Work out the finished part from the listing and answer in its coordinate system (mm). Coordinates: 2 decimals unless noted, no trailing zeros. Loops run counter-clockwise (first coordinate to the right, second up) from the corner with the lowest first, then second, coordinate; pieces in that order, holes last. Notation, with made-up numbers: (-27.5, 85.25) - (30.5, 85.25) arc R29 cw to (30.5, 120.25) - close; hole circle Ø3 at (87.25, 59.5). An arc over 180 degrees is marked (long way). Write each question's results on one line, items separated by ' | '. Start each with the question number.
Item 1: Section B-B, the plane x = 53 is taken. Write down the section's boundary in (y, z), plus the area to 3 significant figures.
Item 2: Each of these flat-tipped pins is pushed along its axis until it touches: pin 1 Ø3.5 at (x, z) = (21.35, -38.1) entering from -Y; pin 2 Ø3 at (y, z) = (2, -113) entering from +X. Where does it stop, or does it pass through?
Item 3: Consider probe 1 along Z at (x, y) = (42, 0.5) (3 decimals); probe 2 along Z at (x, y) = (40.4, 4.5) (3 decimals); probe 3 along X at (y, z) = (4, -38.1). Determine where each line is inside the solid, lowest interval first. Write a range as [from, to].
Item 4: Section A-A, the plane z = -337.5 is taken. Write down the section's boundary in (x, y).
from build123d import *

# Parameters (mm, degrees)
BOSS_EXTRUDE1_DEPTH          = 6.35
F_4_0_4_DIAMETER_HOLE1_D     = 4
F_4_0_4_DIAMETER_HOLE1_DEPTH = 10
F_4_0_4_DIAMETER_HOLE1_TIP   = 1.201721238
F_4_0_4_DIAMETER_HOLE2_D     = 4
F_4_0_4_DIAMETER_HOLE2_DEPTH = 10
F_4_0_4_DIAMETER_HOLE2_TIP   = 1.201721238


with BuildPart() as part:
    # Sketch1 → Boss-Extrude1 (new body)
    with BuildSketch(Plane(origin=(0, 0, 0), x_dir=(1, 0, 0), z_dir=(0, 1, 0))):
        Polygon((0, 0), (216.51, 0), (0, 375), align=None)
    extrude(amount=BOSS_EXTRUDE1_DEPTH)

    # Ø4.0 (4) Diameter Hole1
    with Locations(Plane(origin=(31.757248956, 6.35, -326.345678088), x_dir=(0.50000632, 0, 0.866021755), z_dir=(0, 1, 0))):
        with Locations((21.272379971, -34.925), (40.322379971, -12.7), (244.423337674, -153.137564848), (273.195791575, -147.752490889)):
            Hole(F_4_0_4_DIAMETER_HOLE1_D / 2, depth=F_4_0_4_DIAMETER_HOLE1_DEPTH)
            with Locations((0, 0, -(F_4_0_4_DIAMETER_HOLE1_DEPTH + F_4_0_4_DIAMETER_HOLE1_TIP / 2))):  # 118° drill point
                Cone(0, F_4_0_4_DIAMETER_HOLE1_D / 2, F_4_0_4_DIAMETER_HOLE1_TIP, mode=Mode.SUBTRACT)

    # Ø4.0 (4) Diameter Hole2
    with Locations(Plane(origin=(31.757248956, 0, -326.345678088), x_dir=(-0.50000632, 0, -0.866021755), z_dir=(0, -1, 0))):
        with Locations((-21.272379971, -12.7), (-40.322379971, -34.925), (-253.948458076, -136.639850421), (-263.670671173, -164.250205317)):
            Hole(F_4_0_4_DIAMETER_HOLE2_D / 2, depth=F_4_0_4_DIAMETER_HOLE2_DEPTH)
            with Locations((0, 0, -(F_4_0_4_DIAMETER_HOLE2_DEPTH + F_4_0_4_DIAMETER_HOLE2_TIP / 2))):  # 118° drill point
                Cone(0, F_4_0_4_DIAMETER_HOLE2_D / 2, F_4_0_4_DIAMETER_HOLE2_TIP, mode=Mode.SUBTRACT)


solid = part.part
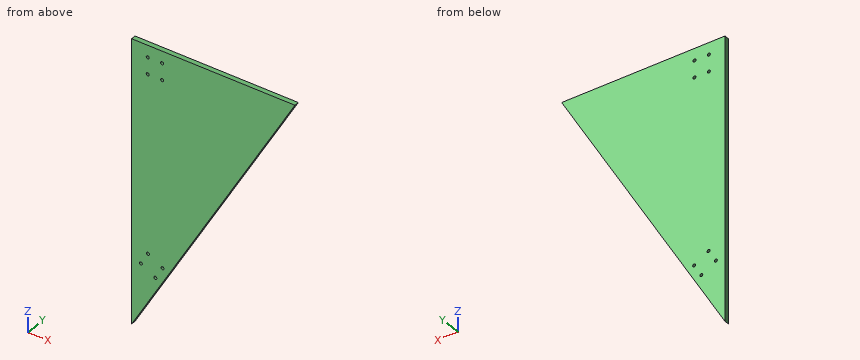
Answer key:
1) outline: (0, -283.2) - (6.35, -283.2) - (6.35, 0) - (0, 0) - close | area: 1,800 mm^2
2) pin 1: passes through | pin 2: stops at x = 152.13
3) probe 1: z = [-302.255, -286.759], [-283.392, -39.3], [-36.9, -17.075], [-14.675, 0] | probe 2: z = [-305.026, -287.007], [-283.144, -40.1], [-36.1, -17.875], [-13.875, 0] | probe 3: x = [0, 19.35], [23.35, 38.4], [42.4, 194.51]
4) outline: (0, 0) - (21.65, 0) - (21.65, 6.35) - (0, 6.35) - close
